Could you check a few things on this model? Use its own coordinates, in mm. Give positions to 0.01 mm unless a question says otherwise; leave off trailing zeros. Write each loop counter-clockwise with the first axis right and the second up, starting at its lowest first coordinate (ties: lowest second). Pieces come first, ordered by that corner, then holes. Notation, with made-up numbers: M 0.25,66 L 54.25,66 A25 ccw 54.25,93 Z; hole C 49,32 d5. An arc over 180 degrees is marked long. Use one line per item in the form item = value.
from build123d import *

# Parameters (mm, degrees)
F0_W     = 29.0246267504
F0_H     = 60
F1_DEPTH = 25.4
F2_SIZE  = 10.16
F4_D     = 5
F5_R     = 1


with BuildPart() as f1:
    # F0 (on Top) → F1 (new body)
    with BuildSketch(Plane.XY):
        with Locations((-14.5123133752, 30)):
            Rectangle(F0_W, F0_H)
    extrude(amount=F1_DEPTH)

    # F2
    f2_edges = [f1.edges().sort_by_distance(p)[0] for p in [
        (0, 30, 25.4),
    ]]
    chamfer(f2_edges, length=F2_SIZE)

    # F4 (through all)
    with Locations(Plane(origin=(7.62, 0, 7.62), x_dir=(0, 1, 0), z_dir=(0.7071067812, 0, 0.7071067812))):
        with Locations((13.411517255, 18.3293204755), (31.2496982515, 18.3293204755)):
            Hole(F4_D / 2)

    # F5
    f5_edges = [f1.edges().sort_by_distance(p)[0] for p in [
        (-14.512313, 60, 0),
    ]]
    fillet(f5_edges, radius=F5_R)


solid = f1.part
1) For pin 1 Ø1.5 at (y, z) = (28, 20) entering from +X, with a flat end and sliding along its axis, tell me the tip position at first contact or that it passes through.
Checked values:
pin_1 = -4.01
2) I want a section at B-B, the plane x = -22. Count the separate pieces of the cut face and the enclosed holes in it, plus the area to 3 significant figures.
Checked values:
separate_pieces = 1
enclosed_holes = 2
area = 1,470 mm2
3) If I drill on L1, parallel to Y at x = -10, z = 15.25; L2, parallel to Y at x = -14.75, z = 10.25; L3, parallel to X at y = 38.5, z = 15.25, over which ranges is the centre line in solid material (lowest first)?
Checked values:
L1 = 0 to 10.96, 15.87 to 28.8, 33.7 to 60
L2 = 0 to 11, 15.83 to 28.84, 33.66 to 60
L3 = -29.02 to -0.01
4) I want a section at A-A, the plane y = 41. Please give me the cut outline in (x, z).
Checked values:
outline = M -29.02,0 L 0,0 L 0,15.24 L -10.16,25.4 L -29.02,25.4 Z
5) Thinking about a two-plate mould opening in X: for faces 1 (the cylindrical face through (-18.052, 12.068, 10.85)), 2 (the flat face through (-29.025, 30, 13)), 3 (the cylindrical face through (-18.052, 29.906, 10.85)), 4 (the flat face through (-20, 30, 25.4)), which applies, released by +X, released by -X, zero draft, split by the parting line, or undercut?
Checked values:
face_1 = undercut
face_2 = released by -X
face_3 = undercut
face_4 = zero draft
